```python
from build123d import *

# Parameters (mm, degrees)
RESSALTO_EXTRUS_O1_DEPTH = 10
ESBO_O2_R                = 1.65
CORTE_EXTRUS_O1_DEPTH    = 15


with BuildPart() as part:
    # Esboço1 → Ressalto-extrusão1 (new body, symmetric)
    with BuildSketch(Plane.XY):
        Polygon((-1.5, 0), (-14, 0), (-14, 6), (14, 6), (14, 0), (1.5, 0), (0, 1), align=None)
    extrude(amount=RESSALTO_EXTRUS_O1_DEPTH, both=True)

    # Esboço2 → Corte-extrusão1 (cut)
    with BuildSketch(Plane.XZ):
        with Locations((-9, 0)):
            Circle(ESBO_O2_R)
        with Locations((9, 0)):
            Circle(ESBO_O2_R)
    extrude(amount=-CORTE_EXTRUS_O1_DEPTH, mode=Mode.SUBTRACT)


solid = part.part
```
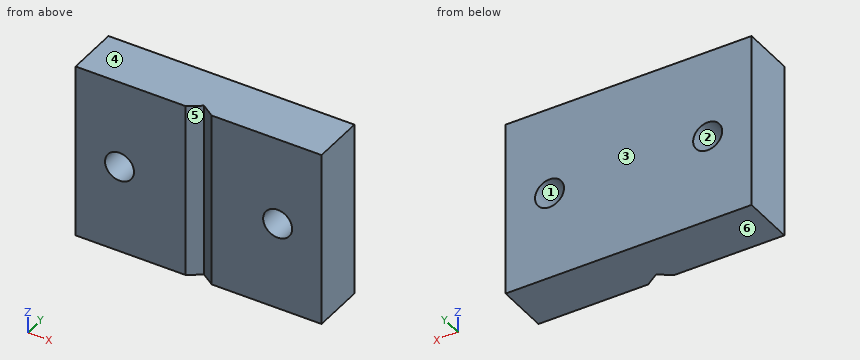
Source: CAD feature listing. Evaluate the final solid. Frame: model axes, mm. Face numbers are marked on the shaded views. A direction names the side the tool comes from. Give positions to 0.01 mm unless a question says otherwise; leave off trailing zeros. Loops run counter-clockwise (first coordinate to the right, second up) from the corner with the lowest first, then second, coordinate; pieces in that order, holes last. Notation, with made-up numbers: (72.25, 17) - (85.25, 17) arc R17 ccw to (85.25, 26) - close; hole circle Ø5 at (-20.75, 44). An arc over 180 degrees is marked (long way). Use CSV: the item, a comma, the result in double quotes.
1) Pin query (flat end, axial travel): P1, Ø5, axis at x = -7, z = -2, coming from the -Y side; P2, Ø2, axis at x = 9, z = 0, coming from the +Y side. Return the tip coordinate at first contact, or that it passes through.
Worked out:
P1,"stops at y = 0"
P2,"passes through"
2) Cut plane A-A (x = -9). Output: boundary loops of the cut face in (y, z), and give its area (3 significant figures).
Worked out:
outline,"(0, -10) - (6, -10) - (6, -1.65) - (0, -1.65) - close; (0, 1.65) - (6, 1.65) - (6, 10) - (0, 10) - close"
area,"100 mm^2"
3) Mould query, pull axis Z, two halves, no side actions, for the marked faces 1, 2, 3 and 4. Classes: +Z half, -Z half, draft (parallel to the pull), parting line (faces both ways), or undercut.
Worked out:
face 1,"undercut"
face 2,"undercut"
face 3,"draft"
face 4,"+Z half"
4) Cut plane D-D (x = 0.75). Output: boundary loops of the cut face in (y, z).
Worked out:
outline,"(0.5, -10) - (6, -10) - (6, 10) - (0.5, 10) - close"
5) Set-up query: the marked faces 5 and 6. Return all of +Z, -Z, +X, -X, +Y, -Y with unobstructed straight access to the full face (end or side cutting, diameter ignored); none if empty.
Worked out:
face 5,"+Z, -Z, -Y"
face 6,"-Z, +X, -X, +Y, -Y"
6) Cut plane C-C (y = 4.85). Output: boundary loops of the cut face in (x, z).
Worked out:
outline,"(-14, -10) - (14, -10) - (14, 10) - (-14, 10) - close; hole circle Ø3.3 at (-9, 0); hole circle Ø3.3 at (9, 0)"
7) Line query: line 1 (Z direction, x = -9, y = 4.1); line 2 (X direction, y = 0.4, z = -7.25); line 3 (Z direction, x = -10, y = 5.35). Output: solid intervals per line, ascending.
Worked out:
line 1,"z = -10 to -1.65, 1.65 to 10"
line 2,"x = -14 to -0.9, 0.9 to 14"
line 3,"z = -10 to -1.31, 1.31 to 10"
8) Cut plane B-B (z = 0). Output: boundary loops of the cut face in (x, y).
Worked out:
outline,"(-14, 0) - (-10.65, 0) - (-10.65, 6) - (-14, 6) - close; (-7.35, 0) - (-1.5, 0) - (0, 1) - (1.5, 0) - (7.35, 0) - (7.35, 6) - (-7.35, 6) - close; (10.65, 0) - (14, 0) - (14, 6) - (10.65, 6) - close"
